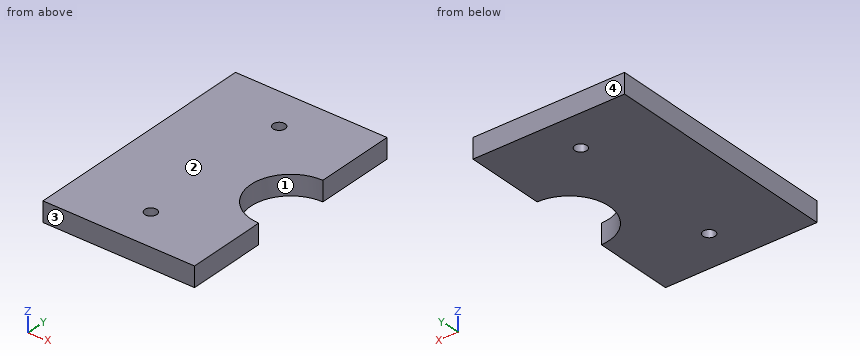
from build123d import *

# Parameters (mm, degrees)
SKETCH_1_W          = 75.760831706
SKETCH_1_H          = 120
SKETCH_1_R          = 3
EXTRUDE_1_DEPTH     = 10
SKETCH_5_R          = 20
CUT_EXTRUDE_1_DEPTH = 20


with BuildPart() as part:
    # 草图1 → 凸台-拉伸1 (new body)
    # profile 1 of 2: a face of its own
    with BuildSketch(Plane.XY):
        with BuildLine():
            Line((0, -37.880415853), (0, 37.880415853))
            ThreePointArc((0, 37.880415853), (-37.880415853, 0), (0, -37.880415853))
        make_face()
    # profile 2 of 2: a face of its own
    with BuildSketch(Plane.XY):
        with Locations((-37.880415853, 0)):
            Rectangle(SKETCH_1_W, SKETCH_1_H)
        with Locations((-37.880415853, -40)):
            Circle(SKETCH_1_R, mode=Mode.SUBTRACT)
        with Locations((-37.880415853, 40)):
            Circle(SKETCH_1_R, mode=Mode.SUBTRACT)
    extrude(amount=EXTRUDE_1_DEPTH)

    # 草图5 → 切除-拉伸1 (cut)
    with BuildSketch(Plane.XY.offset(10)):
        Circle(SKETCH_5_R)
    extrude(amount=-CUT_EXTRUDE_1_DEPTH, mode=Mode.SUBTRACT)


solid = part.part
Geometry check sheet. Reference: the model listing, model coordinates, mm. Face numbers are marked on the shaded views. Round coordinates to 2 decimals unless told otherwise and drop trailing zeros. Order: outer loops, then holes, each group sorted by start corner. A loop starts at its lowest first (then second) coordinate and runs counter-clockwise, first axis right, second up. Notation, with made-up numbers: M 12,-8.5 L 50,-8.5 A29 cw 50,16.5 Z; hole C 37,19.5 d7. An arc over 180 degrees is marked long. Write each question's results on one line, items separated by ' | '. Start each with the question number.
1. Cross-section at D-D on y = 0. Record the boundary of the cut face in (x, z), plus the area to 3 significant figures.
2. Cross-section at A-A on y = 40. Record the boundary of the cut face in (x, z).
3. Cross-section at C-C on z = 8. Record the boundary of the cut face in (x, y).
4. Draft check along Y on the marked faces 1, 2, 3 and 4. Enter one of: pulls with the +Y half, pulls with the -Y half, needs draft (parallel to the pull), parting line crosses it, or undercut.
5. Material ranges on L1, parallel to Y at x = -37.5, z = 3.5; L2, parallel to Y at x = -8, z = 7.5; L3, parallel to Y at x = -7.5, z = 4.5, recorded low to high. Write a range as from..to.
6. Cross-section at B-B on x = -4.5. Record the boundary of the cut face in (y, z), plus the area to 3 significant figures.
7. Go/stop test with flat-tipped pins: P1, Ø1, axis at y = 4.5, z = 5.5, coming from the +X side; P2, Ø3.5, axis at x = -37.88, y = 40, coming from the -Z side; P3, Ø8, axis at x = -37.88, y = -40, coming from the -Z side; P4, Ø5, axis at y = 9, z = 6, coming from the +X side. Record where each tip stops, or that it passes through.
Resolved:
1) outline: M -75.76,0 L -20,0 L -20,10 L -75.76,10 Z | area: 558 mm2
2) outline: M -75.76,0 L -40.88,0 L -40.88,10 L -75.76,10 Z; M -34.88,0 L 0,0 L 0,10 L -34.88,10 Z
3) outline: M -75.76,-60 L 0,-60 L 0,-20 A20 cw 0,20 L 0,60 L -75.76,60 Z; hole C -37.88,-40 d6; hole C -37.88,40 d6
4) face 1: undercut | face 2: needs draft | face 3: pulls with the -Y half | face 4: pulls with the +Y half
5) L1: -60..-42.98, -37.02..37.02, 42.98..60 | L2: -60..-18.33, 18.33..60 | L3: -60..-18.54, 18.54..60
6) outline: M -60,0 L -19.49,0 L -19.49,10 L -60,10 Z; M 19.49,0 L 60,0 L 60,10 L 19.49,10 Z | area: 810 mm2
7) P1: x = -19.36 | P2: through | P3: z = 0 | P4: x = -16.36
